Design review of the part built by this model. Coordinates are the model's own, in mm. A direction names the side the tool comes from. Coordinates: 2 decimals unless noted, no trailing zeros. Write each loop counter-clockwise with the first axis right and the second up, starting at its lowest first coordinate (ties: lowest second). Pieces come first, ordered by that corner, then holes.
Q1. Machinability: for faces 1 (the flat face through (4, 27, 8)), 2 (the flat face through (4, 55.6, 2)), 3 (the flat face through (4, 8, 6)), which of the approach directions +Z, -Z, +X, -X, +Y, -Y give a long, thin tool a straight path to every point of the face, cutting with its end or side? Answer none if there is none.
Q2. Insertion check: pin 1 (3.5 mm diameter, centred on x = 3.5, z = 3, fed in from -Y); pin 2 (1 mm diameter, centred on y = 17, z = 3.5, fed in from -X); pin 3 (2 mm diameter, centred on x = 3.5, z = 0.5, fed in from +Y). Each pin has a flat end and moves straight along its axis. Give the tip position at first contact, or say it passes through.
Q3. Take a section at A-A (y = 32.5). Give the boundary of the cut face in (x, z), and give its area (3 significant figures).
Q4. Take a section at B-B (z = 0). Give the boundary of the cut face in (x, y), and give its area (3 significant figures).
Q5. For probe 1 along Z at (x, y) = (6.5, 40); probe 2 along Y at (x, z) = (4.25, -0.25); probe 3 along Z at (x, y) = (4.5, 47), list the stretches that pass through material, from the lowest coordinate up.
```python
from build123d import *

# Parameters (mm, degrees)
BOSS_EXTRUDE1_DEPTH = 8
BOSS_EXTRUDE2_DEPTH = 8
BOSS_EXTRUDE4_DEPTH = 8
SKETCH10_W          = 4.468992015
SKETCH10_H          = 1.428902643
CUT_EXTRUDE2_DEPTH  = 2
SKETCH11_W          = 1.778541799
SKETCH11_H          = 8.6
SKETCH11_W_2        = 1.752466186
CUT_EXTRUDE4_DEPTH  = 2.5
CUT_EXTRUDE6_DEPTH  = 14.47


with BuildPart() as part:
    # Sketch2 → Boss-Extrude1 (new body)
    with BuildSketch(Plane.YZ):
        with BuildLine():
            Line((55, 6), (0, 6))
            ThreePointArc((0, 6), (-6, 0), (0, -6))
            Line((0, -6), (55, -6))
            Line((55, -6), (55, -8))
            Line((55, -8), (0, -8))
            ThreePointArc((0, -8), (-8, 0), (0, 8))
            Line((0, 8), (55, 8))
            Line((55, 8), (55, 6))
        make_face()
    extrude(amount=BOSS_EXTRUDE1_DEPTH)

    # Sketch8 → Boss-Extrude2 (add)
    with BuildSketch(Plane.YZ):
        Polygon((8.883709987, 6.2), (11.885253021, 6.2), (10.384481504, 5.074983791), align=None)
        Polygon((4.883709987, 6.2), (7.885253021, 6.2), (6.384481504, 5.074983791), align=None)
        Polygon((12.883709987, 6.2), (15.885253021, 6.2), (14.384481504, 5.074983791), align=None)
        Polygon((16.883709987, 6.2), (19.885253021, 6.2), (18.384481504, 5.074983791), align=None)
        Polygon((20.883709987, 6.2), (23.885253021, 6.2), (22.384481504, 5.074983791), align=None)
        Polygon((24.883709987, 6.2), (27.885253021, 6.2), (26.384481504, 5.074983791), align=None)
        Polygon((28.883709987, 6.2), (31.885253021, 6.2), (30.384481504, 5.074983791), align=None)
        Polygon((32.883709987, 6.2), (35.885253021, 6.2), (34.384481504, 5.074983791), align=None)
        Polygon((36.883709987, 6.2), (39.885253021, 6.2), (38.384481504, 5.074983791), align=None)
        Polygon((40.883709987, 6.2), (43.885253021, 6.2), (42.384481504, 5.074983791), align=None)
        Polygon((44.883709987, 6.2), (47.885253021, 6.2), (46.384481504, 5.074983791), align=None)
        Polygon((48.883709987, 6.2), (51.885253021, 6.2), (50.384481504, 5.074983791), align=None)
    boss_extrude2 = extrude(amount=BOSS_EXTRUDE2_DEPTH)

    # Mirror1: Boss-Extrude2 across plane
    add(boss_extrude2.mirror(Plane.XY))

    # Sketch9 → Boss-Extrude4 (add)
    with BuildSketch(Plane.YZ):
        Polygon((55, 6), (55, -2), (53.75, -2), (53.75, -1.5), (53.25, -1.5), (53.25, -2), (53.25, -2.6), (55.6, -2.6), (55.6, 6), (56.503482489, 6), (55, 8), align=None)
        Polygon((53.75, -4.000391414), (51.384098648, -6), (53.75, -6), align=None)
    extrude(amount=BOSS_EXTRUDE4_DEPTH)

    # Sketch10 → Cut-Extrude2 (cut)
    with BuildSketch(Plane(origin=(0, 53.75, 0), x_dir=(-1, 0, 0), z_dir=(0, 1, 0))):
        with Locations((-3.986962194, -5.0167747)):
            Rectangle(SKETCH10_W, SKETCH10_H)
    extrude(amount=-CUT_EXTRUDE2_DEPTH, mode=Mode.SUBTRACT)

    # Sketch11 → Cut-Extrude4 (cut)
    with BuildSketch(Plane(origin=(0, 55.6, 0), x_dir=(-1, 0, 0), z_dir=(0, 1, 0))):
        with Locations((-7.110729101, 1.7)):
            Rectangle(SKETCH11_W, SKETCH11_H)
        with Locations((-0.876233093, 1.7)):
            Rectangle(SKETCH11_W_2, SKETCH11_H)
    extrude(amount=-CUT_EXTRUDE4_DEPTH, mode=Mode.SUBTRACT)

    # Sketch12 → Cut-Extrude6 (cut)
    with BuildSketch(Plane(origin=(1.752466186, 0, 0), x_dir=(0, -1, 0), z_dir=(-1, 0, 0))):
        Polygon((-53.25, -2.6), (-53.25, -2.199701503), (-54.173023817, -2.6), (-53.75, -2.6), align=None)
    extrude(amount=-CUT_EXTRUDE6_DEPTH, mode=Mode.SUBTRACT)


solid = part.part
```
Response:
1. face 1: +Z, +X, -X, +Y, -Y
1. face 2: -Z, +X, -X, +Y
1. face 3: +X, -X
2. pin 1: stops at y = -7.9
2. pin 2: passes through
2. pin 3: stops at y = 55.6
3. outline: (0, -8) - (8, -8) - (8, -6) - (0, -6) - close; (0, 6) - (8, 6) - (8, 8) - (0, 8) - close
3. area: 32.0 mm2
4. outline: (0, -8) - (8, -8) - (8, -6) - (0, -6) - close; (1.75, 55) - (6.22, 55) - (6.22, 55.6) - (1.75, 55.6) - close
4. area: 18.7 mm2
5. probe 1: z = -8 to -6, 6 to 8
5. probe 2: y = -8 to -5.99, 55 to 55.6
5. probe 3: z = -8 to -5.54, 5.54 to 8
